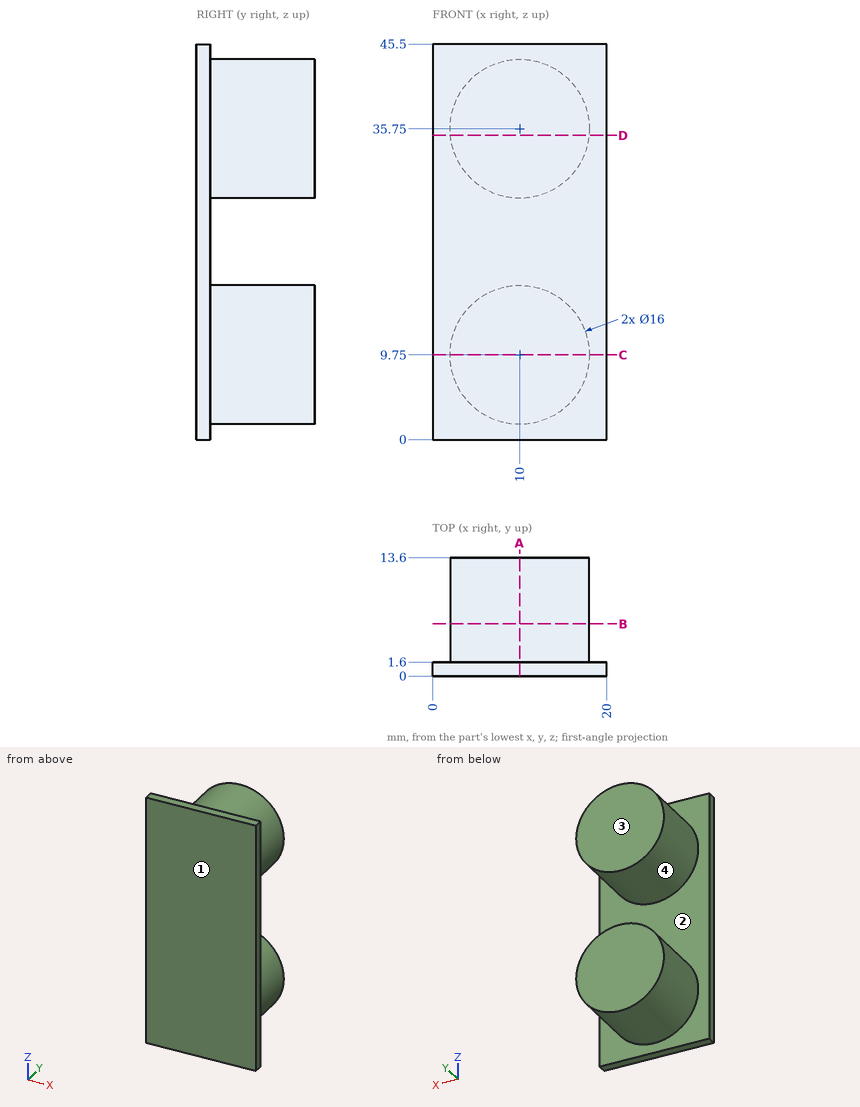
Geometry: see drawing. Coordinates: mm, zero at the bounding-box minimum. A direction names the side the tool comes from. Coordinates: 2 decimals unless noted, no trailing zeros. Loops run counter-clockwise (first coordinate to the right, second up) from the corner with the lowest first, then second, coordinate; pieces in that order, holes last.
Q1. Draft query along Z for the marked faces 1 and 2. Return one class per face: +Z half, -Z half, draft (parallel to the pull), parting line (faces both ways), or undercut.
Q2. Set-up query: the marked faces 3 and 4. Return all of +Z, -Z, +X, -X, +Y, -Y with unobstructed straight access to the full face (end or side cutting, diameter ignored); none if empty.
Q3. Cut plane C-C (z = 9.75). Output: boundary loops of the cut face in (x, y).
Q4. Cut plane A-A (x = 10). Output: boundary loops of the cut face in (y, z).
Q5. Material intervals for line 1 (Y direction, x = 2, z = 14); line 2 (X direction, y = 3, z = 36); line 3 (Z direction, x = 12.5, y = 7.25), sorted ascending.
Q6. Cut plane D-D (z = 35). Output: boundary loops of the cut face in (x, y).
Q7. Cut plane B-B (y = 6). Output: boundary loops of the cut face in (x, z), then the cut area to 3 significant figures.
Q8. Contact query for flat-ended pins moving along their axis: pin 1 (1.5 mm diameter, centred on y = 11, z = 28, fed in from +X); pin 2 (1 mm diameter, centred on y = 5, z = 36, fed in from +X). Output: stop coordinate, or through.
Working result:
1. face 1: draft
1. face 2: undercut
2. face 3: +Z, -Z, +X, -X, +Y
2. face 4: +Y
3. outline: (0, 0) - (20, 0) - (20, 1.6) - (18, 1.6) - (18, 13.6) - (2, 13.6) - (2, 1.6) - (0, 1.6) - close
4. outline: (0, 0) - (1.6, 0) - (1.6, 1.75) - (13.6, 1.75) - (13.6, 17.75) - (1.6, 17.75) - (1.6, 27.75) - (13.6, 27.75) - (13.6, 43.75) - (1.6, 43.75) - (1.6, 45.5) - (0, 45.5) - close
5. line 1: y = 0 to 1.6
5. line 2: x = 2 to 18
5. line 3: z = 2.15 to 17.35, 28.15 to 43.35
6. outline: (0, 0) - (20, 0) - (20, 1.6) - (17.96, 1.6) - (17.96, 13.6) - (2.04, 13.6) - (2.04, 1.6) - (0, 1.6) - close
7. outline: circle Ø16 at (10, 9.75); circle Ø16 at (10, 35.75)
7. area: 402 mm2
8. pin 1: stops at x = 13.87
8. pin 2: stops at x = 18
